Design review of the part built by this model. Coordinates are the model's own, in mm. A direction names the side the tool comes from. Coordinates: 2 decimals unless noted, no trailing zeros. Return JSON: item names as keys, results as strings. Group by question number.
from build123d import *

# Parameters (mm, degrees)
HOLE_WIZARD_M61_D           = 6.4
HOLE_WIZARD_M61_CBORE_D     = 11
HOLE_WIZARD_M61_CBORE_DEPTH = 6.8
SKETCH_4_OUTSIDE_W          = 124.038
SKETCH_4_OUTSIDE_H          = 124.038
CUT_EXTRUDE_1_DEPTH         = 16
SKETCH_5_R                  = 31
CUT_EXTRUDE_2_DEPTH         = 1.5
FILLET_1_R                  = 0.6
FILLET_2_R                  = 0.5
FILLET_3_R                  = 0.6


with BuildPart() as part:
    # Эскиз1 → Повернуть1 (revolve)
    with BuildSketch(Plane.XY):
        Polygon((-4.5, 23), (-2.736707365, 23), (-2, 29), (2, 29), (2.736707365, 23), (4.5, 23), (4.5, 28), (10.5, 28), (10.5, 31), (5.5, 31), (5.5, 47.5), (-4.5, 47.5), align=None)
    revolve(axis=Axis((0, 0, 0), (1, 0, 0)))

    # Цековка для  болта с шестигранной головкой M61 (through all)
    with Locations(Plane(origin=(-4.5, 27.577164466, -27.577164466), x_dir=(0, 0, -1), z_dir=(-1, 0, 0))):
        with Locations((0, 0), (-55.154328932, 0), (-55.154328932, 55.154328932), (0, 55.154328932)):
            CounterBoreHole(HOLE_WIZARD_M61_D / 2, HOLE_WIZARD_M61_CBORE_D / 2, HOLE_WIZARD_M61_CBORE_DEPTH)

    # Эскиз4 outside → Вытянуть1 (cut, through all)
    with BuildSketch(Plane.ZY.offset(4.5)):
        Rectangle(SKETCH_4_OUTSIDE_W, SKETCH_4_OUTSIDE_H)
        with BuildLine():
            Line((-36.077164466, 27.577164466), (-36.077164466, -27.577164466))
            ThreePointArc((-36.077164466, -27.577164466), (-33.587572106, -33.587572106), (-27.577164466, -36.077164466))
            Line((-27.577164466, -36.077164466), (27.577164466, -36.077164466))
            ThreePointArc((27.577164466, -36.077164466), (33.587572106, -33.587572106), (36.077164466, -27.577164466))
            Line((36.077164466, -27.577164466), (36.077164466, 27.577164466))
            ThreePointArc((36.077164466, 27.577164466), (33.587572106, 33.587572106), (27.577164466, 36.077164466))
            Line((27.577164466, 36.077164466), (-27.577164466, 36.077164466))
            ThreePointArc((-27.577164466, 36.077164466), (-33.587572106, 33.587572106), (-36.077164466, 27.577164466))
        make_face(mode=Mode.SUBTRACT)
    extrude(amount=-CUT_EXTRUDE_1_DEPTH, mode=Mode.SUBTRACT)

    # Эскиз5 → Вытянуть2 (cut)
    with BuildSketch(Plane(origin=(10.5, 0, 0), x_dir=(0, 0, -1), z_dir=(1, 0, 0))):
        Circle(SKETCH_5_R)
    extrude(amount=-CUT_EXTRUDE_2_DEPTH, mode=Mode.SUBTRACT)

    # Скругление1
    fillet_1_edges = [part.edges().sort_by_distance(p)[0] for p in [
        (5.5, -31, 0),
    ]]
    fillet(fillet_1_edges, radius=FILLET_1_R)

    # Скругление2
    fillet_2_edges = [part.edges().sort_by_distance(p)[0] for p in [
        (9, -31, 0),
        (9, -28, 0),
    ]]
    fillet(fillet_2_edges, radius=FILLET_2_R)

    # Скругление3
    fillet_3_edges = [part.edges().sort_by_distance(p)[0] for p in [
        (4.5, -28, 0),
    ]]
    fillet(fillet_3_edges, radius=FILLET_3_R)


solid = part.part
Item 1: For P1, Ø7.5, axis at y = 27.58, z = 27.58, coming from the +X side; P2, Ø5.5, axis at y = 25.5, z = -25.5, coming from the -X side; P3, Ø8.5, axis at y = 27.58, z = -27.58, coming from the -X side, all flat-tipped, find the tip position at first contact; note any pin that passes through.
Item 2: To check wall thickness, follow line 1 (Y direction, x = 0.5, z = -24); line 2 (Y direction, x = -2.75, z = 25); line 3 (Y direction, x = 1.5, z = -7.5). State the ranges of each line that lie inside material, in increasing order. Write a range as from..to.
Item 3: For faces 1 (the face through (0.03, 13.38, -25.73)), 2 (the face through (6.824, 25.865, -10.724)), 3 (the face through (0.43, 33.521, 33.653)), 4 (the face through (-3.606, -2.994, 22.804)), 5 (the face through (2.3, 30, -30)), list the 3-axis set-ups (+Z, -Z, +X, -X, +Y, -Y) from which the entire face can be reached by the end or side of a thin tool; tool diameter is ignored.
Item 4: Draft analysis for pull direction Z (two halves, no side actions). For faces 6 (the face through (0.43, 33.653, -33.521)), 7 (the face through (0, 0, 36.077)), 8 (the face through (-1.148, -27.819, -22.082)), state which applies: pulls with the +Z half, pulls with the -Z half, needs draft (parallel to the pull), parting line crosses it, or undercut.
Answers below:
{
 "1": {"P1": "stops at x = 5.5", "P2": "stops at x = -4.5", "P3": "stops at x = 2.3"},
 "2": {"line 1": "y = -36.08..-31.75, -23.4..-16.28, 16.28..23.4, 31.75..36.08", "line 2": "y = -36.08..-32.44, -22.72..22.72, 32.44..36.08", "line 3": "y = -36.08..-28.01, 28.01..36.08"},
 "3": {"face 1": "none", "face 2": "+X", "face 3": "+Z, +X, -X, +Y", "face 4": "+X, -X", "face 5": "-X"},
 "4": {"face 6": "pulls with the -Z half", "face 7": "pulls with the +Z half", "face 8": "undercut"}
}
